Read the model definition and answer for the solid it produces. Units are mm, in the model's axes. A direction names the side the tool comes from. Coordinates: 2 decimals unless noted, no trailing zeros. Write each loop counter-clockwise with the first axis right and the second up, starting at its lowest first coordinate (ties: lowest second). Pieces come first, ordered by that corner, then holes.
(1) Straight lines are drawn through the part: line 1 along Y through (x, z) = (14, 0); line 2 along Z through (x, y) = (7.5, 4.25); line 3 along Z through (x, y) = (10.5, 1.5). For each, find the intervals that lie inside material, in ascending order.
(2) The part is cut by section A-A, the plane z = 0. Determine the outline of the cut face in (x, y), and give its area (4 significant figures).
(3) The part is cut by section D-D, the plane z = -5.25. Determine the outline of the cut face in (x, y).
(4) The part is cut by section B-B, the plane x = -14. Determine the outline of the cut face in (y, z), and give its area (4 significant figures).
(5) Which of the six approach directions +Z, -Z, +X, -X, +Y, -Y give full straight-line access (tool end or side, diameter ignored) to faces 1 (the flat face through (0, -4, -5)), 2 (the flat face through (0, 4, -5)), 3 (the flat face through (0, 4, 5)), 4 (the cylindrical face through (-13.55, 9.2, 1.43))?
(6) The part is cut by section C-C, the plane y = -2.75. Determine the outline of the cut face in (x, z), and give its area (3 significant figures).
(7) Given pin 1 (2 mm diameter, centred on x = 5, y = -2, fed in from +Z); pin 2 (5 mm diameter, centred on y = 8, z = 2.5, fed in from -X); pin 3 (1.5 mm diameter, centred on x = -7.5, z = 1, fed in from +Y), each flat-ended and moving along its own axis, determine where each tip first touches the part or whether it passes through.
```python
from build123d import *

# Parameters (mm, degrees)
BOSS_EXTRUDE1_DEPTH = 15.1
BOSS_EXTRUDE2_START = -18
BOSS_EXTRUDE2_DEPTH = 18
BOSS_EXTRUDE3_START = 5
SKETCH2_R           = 1.5
BOSS_EXTRUDE3_DEPTH = 8
BOSS_EXTRUDE4_START = 5
SKETCH2_3_R         = 2
SKETCH2_3_R_2       = 1.5
BOSS_EXTRUDE4_DEPTH = 0.5


with BuildPart() as part:
    # Sketch1 → Boss-Extrude1 (new body)
    with BuildSketch(Plane(origin=(0, 0, 0), x_dir=(0, 0, -1), z_dir=(1, 0, 0))):
        with BuildLine():
            Line((3.31662479, 5), (-3.31662479, 5))
            ThreePointArc((-3.31662479, 5), (-5.286764074, 2.837274331), (-6, 0))
            ThreePointArc((-6, 0), (-5.286764074, -2.837274331), (-3.31662479, -5))
            Line((-3.31662479, -5), (3.31662479, -5))
            ThreePointArc((3.31662479, -5), (5.286764074, -2.837274331), (6, 0))
            ThreePointArc((6, 0), (5.286764074, 2.837274331), (3.31662479, 5))
        make_face()
    extrude(amount=BOSS_EXTRUDE1_DEPTH)

    # Sketch1<3> → Boss-Extrude2 (add)
    with BuildSketch(Plane(origin=(0, 0, 0), x_dir=(0, 0, -1), z_dir=(1, 0, 0)).offset(BOSS_EXTRUDE2_START)):
        with BuildLine():
            Line((-3.31662479, 5), (-6, 5))
            Line((-6, 5), (-6, 0))
            ThreePointArc((-6, 0), (-5.286764074, 2.837274331), (-3.31662479, 5))
        make_face()
        with BuildLine():
            Line((3.31662479, 5), (-3.31662479, 5))
            ThreePointArc((-3.31662479, 5), (-5.286764074, 2.837274331), (-6, 0))
            ThreePointArc((-6, 0), (-5.286764074, -2.837274331), (-3.31662479, -5))
            Line((-3.31662479, -5), (3.31662479, -5))
            ThreePointArc((3.31662479, -5), (5.286764074, -2.837274331), (6, 0))
            ThreePointArc((6, 0), (5.286764074, 2.837274331), (3.31662479, 5))
        make_face()
        with BuildLine():
            Line((6, 5), (3.31662479, 5))
            ThreePointArc((3.31662479, 5), (5.286764074, 2.837274331), (6, 0))
            Line((6, 0), (6, 5))
        make_face()
        with BuildLine():
            ThreePointArc((-3.31662479, -5), (-5.286764074, -2.837274331), (-6, 0))
            Line((-6, 0), (-6, -5))
            Line((-6, -5), (-3.31662479, -5))
        make_face()
        with BuildLine():
            Line((6, -5), (6, 0))
            ThreePointArc((6, 0), (5.286764074, -2.837274331), (3.31662479, -5))
            Line((3.31662479, -5), (6, -5))
        make_face()
    extrude(amount=BOSS_EXTRUDE2_DEPTH)

    # Sketch2 → Boss-Extrude3 (add)
    with BuildSketch(Plane(origin=(0, 0, 0), x_dir=(1, 0, 0), z_dir=(0, 1, 0)).offset(BOSS_EXTRUDE3_START)):
        with Locations(Location((-14, 0, 0), (0, 0, 270))):
            Circle(SKETCH2_R)
    extrude(amount=BOSS_EXTRUDE3_DEPTH)

    # Sketch2<3> → Boss-Extrude4 (add)
    with BuildSketch(Plane(origin=(0, 0, 0), x_dir=(1, 0, 0), z_dir=(0, 1, 0)).offset(BOSS_EXTRUDE4_START)):
        with Locations(Location((-14, 0, 0), (0, 0, 270))):
            Circle(SKETCH2_3_R)
        with Locations(Location((-14, 0, 0), (0, 0, 270))):
            Circle(SKETCH2_3_R_2, mode=Mode.SUBTRACT)
    extrude(amount=BOSS_EXTRUDE4_DEPTH)


solid = part.part
```
Computed:
1. line 1: y = -5 to 5
1. line 2: z = -4.24 to 4.24
1. line 3: z = -5.81 to 5.81
2. outline: (-18, -5) - (15.1, -5) - (15.1, 5) - (-12, 5) - (-12, 5.5) - (-12.5, 5.5) - (-12.5, 13) - (-15.5, 13) - (-15.5, 5.5) - (-16, 5.5) - (-16, 5) - (-18, 5) - close
2. area: 355.5 mm2
3. outline: (-18, -5) - (0, -5) - (0, -2.9) - (15.1, -2.9) - (15.1, 2.9) - (0, 2.9) - (0, 5) - (-18, 5) - close
4. outline: (-5, -6) - (5, -6) - (5, -2) - (5.5, -2) - (5.5, -1.5) - (13, -1.5) - (13, 1.5) - (5.5, 1.5) - (5.5, 2) - (5, 2) - (5, 6) - (-5, 6) - close
4. area: 144.5 mm2
5. face 1: -Z, +X, -Y
5. face 2: -Z, +X, +Y
5. face 3: +Z, +X, +Y
5. face 4: +Y
6. outline: (-18, -6) - (0, -6) - (0, -5.33) - (15.1, -5.33) - (15.1, 5.33) - (0, 5.33) - (0, 6) - (-18, 6) - close
6. area: 377 mm2
7. pin 1: stops at z = 5.92
7. pin 2: stops at x = -15.5
7. pin 3: stops at y = 5
